```python
from build123d import *

# Parameters (mm, degrees)
F0_W     = 219.9670784175
F0_H     = 257.1922540665
F0_H_2   = 477.1593213081
F0_W_2   = 720.8151631057
F0_H_3   = 247.0399104059
F0_H_4   = 372.2520321608
F1_DEPTH = 635


with BuildPart() as f1:
    # F0 (on Front) → F1 (new body)
    with BuildSketch(Plane.XZ):
        with BuildLine():
            Line((-825.5, -1066.8), (825.5, -1066.8))
            Line((825.5, -1066.8), (825.5, 1016))
            ThreePointArc((825.5, 1016), (810.6210244843, 1051.9210244843), (774.7, 1066.8))
            Line((774.7, 1066.8), (-774.7, 1066.8))
            ThreePointArc((-774.7, 1066.8), (-810.6210244843, 1051.9210244843), (-825.5, 1016))
            Line((-825.5, 1016), (-825.5, -1066.8))
        make_face()
        with BuildLine():
            ThreePointArc((107.7734987259, 1034.2634128571), (109.6333706654, 1038.7535409176), (114.1234987259, 1040.6134128571))
            Line((114.1234987259, 1040.6134128571), (736.4234987259, 1040.6134128571))
            ThreePointArc((736.4234987259, 1040.6134128571), (740.9136267864, 1038.7535409176), (742.7734987259, 1034.2634128571))
            Line((742.7734987259, 1034.2634128571), (742.7734987259, -1035.8365871429))
            ThreePointArc((742.7734987259, -1035.8365871429), (740.9136267864, -1040.3267152035), (736.4234987259, -1042.1865871429))
            Line((736.4234987259, -1042.1865871429), (114.1234987259, -1042.1865871429))
            ThreePointArc((114.1234987259, -1042.1865871429), (109.6333706654, -1040.3267152035), (107.7734987259, -1035.8365871429))
            Line((107.7734987259, -1035.8365871429), (107.7734987259, 1034.2634128571))
        make_face(mode=Mode.SUBTRACT)
        Polygon((-787.4, -1037.2292995453), (-787.4, 1045.5707004547), (-752.9641985893, 1045.5707004547), (-32.1490354836, 1045.5707004547), (0, 1045.5707004547), (0, -1037.2292995453), (-32.1490354836, -1037.2292995453), (-252.1161139011, -1037.2292995453), (-272.5006639957, -1037.2292995453), (-734.9091768265, -1037.2292995453), (-752.9641985893, -1037.2292995453), align=None, mode=Mode.SUBTRACT)
        Polygon((-752.9641985893, 1045.5707004547), (-787.4, 1045.5707004547), (-787.4, -1037.2292995453), (-752.9641985893, -1037.2292995453), (-752.9641985893, -302.8777241707), (-752.9641985893, -59.2219047248), (-752.9641985893, 187.818005681), (-752.9641985893, 560.0700378418), (-752.9641985893, 593.9111113548), (-752.9641985893, 780.0370454788), (-752.9641985893, 813.8781785965), (-752.9641985893, 854.4874191284), (-752.9641985893, 1016.9246196747), align=None)
        with BuildLine():
            Line((-752.9641985893, -302.8777241707), (-752.9641985893, -1037.2292995453))
            Line((-752.9641985893, -1037.2292995453), (-734.9091768265, -1037.2292995453))
            Line((-734.9091768265, -1037.2292995453), (-734.9091768265, -326.3940406799))
            ThreePointArc((-734.9091768265, -326.3940406799), (-733.049304887, -321.9039126194), (-728.5591768265, -320.0440406799))
            Line((-728.5591768265, -320.0440406799), (-278.8506639957, -320.0440406799))
            ThreePointArc((-278.8506639957, -320.0440406799), (-274.3605359352, -321.9039126194), (-272.5006639957, -326.3940406799))
            Line((-272.5006639957, -326.3940406799), (-272.5006639957, -1037.2292995453))
            Line((-272.5006639957, -1037.2292995453), (-252.1161139011, -1037.2292995453))
            Line((-252.1161139011, -1037.2292995453), (-252.1161139011, -560.0699782372))
            Line((-252.1161139011, -560.0699782372), (-252.1161139011, -302.8777241707))
            Line((-252.1161139011, -302.8777241707), (-752.9641985893, -302.8777241707))
        make_face()
        with Locations((-142.1325746924, -431.4738512039)):
            Rectangle(F0_W, F0_H)
        with BuildLine():
            ThreePointArc((-238.722667098, -327.5587750435), (-236.8627951586, -323.068646983), (-232.372667098, -321.2087750435))
            Line((-232.372667098, -321.2087750435), (-50.5582434893, -321.2087750435))
            ThreePointArc((-50.5582434893, -321.2087750435), (-46.0681154287, -323.068646983), (-44.2082434893, -327.5587750435))
            Line((-44.2082434893, -327.5587750435), (-44.2082434893, -532.6683329582))
            ThreePointArc((-44.2082434893, -532.6683329582), (-46.0681154287, -537.1584610188), (-50.5582434893, -539.0183329582))
            Line((-50.5582434893, -539.0183329582), (-232.372667098, -539.0183329582))
            ThreePointArc((-232.372667098, -539.0183329582), (-236.8627951586, -537.1584610188), (-238.722667098, -532.6683329582))
            Line((-238.722667098, -532.6683329582), (-238.722667098, -327.5587750435))
        make_face(mode=Mode.SUBTRACT)
        with Locations((-142.1325746924, -798.6496388912)):
            Rectangle(F0_W, F0_H_2)
        with BuildLine():
            ThreePointArc((-238.722667098, -582.6405478477), (-236.8627951586, -578.1504197872), (-232.372667098, -576.2905478477))
            Line((-232.372667098, -576.2905478477), (-54.0525136352, -576.2905478477))
            ThreePointArc((-54.0525136352, -576.2905478477), (-49.5623855746, -578.1504197872), (-47.7025136352, -582.6405478477))
            Line((-47.7025136352, -582.6405478477), (-47.7025136352, -1017.207305336))
            ThreePointArc((-47.7025136352, -1017.207305336), (-49.5623855746, -1021.6974333965), (-54.0525136352, -1023.557305336))
            Line((-54.0525136352, -1023.557305336), (-232.372667098, -1023.557305336))
            ThreePointArc((-232.372667098, -1023.557305336), (-236.8627951586, -1021.6974333965), (-238.722667098, -1017.207305336))
            Line((-238.722667098, -1017.207305336), (-238.722667098, -582.6405478477))
        make_face(mode=Mode.SUBTRACT)
        Polygon((-752.9641985893, -59.2219047248), (-752.9641985893, -302.8777241707), (-252.1161139011, -302.8777241707), (-32.1490354836, -59.2219047248), align=None)
        with BuildLine():
            Line((-742.5824999809, -286.2870691341), (-742.5824999809, -75.7915718317))
            ThreePointArc((-742.5824999809, -75.7915718317), (-740.7226280415, -71.3014437712), (-736.2324999809, -69.4415718317))
            Line((-736.2324999809, -69.4415718317), (-71.9638137919, -69.4415718317))
            ThreePointArc((-71.9638137919, -69.4415718317), (-66.1611104022, -73.2125926982), (-67.2504119148, -80.0467266755))
            Line((-67.2504119148, -80.0467266755), (-255.8638893667, -288.972406544))
            ThreePointArc((-255.8638893667, -288.972406544), (-257.9887402532, -290.5156914705), (-260.5563342855, -291.0672171179))
            Line((-260.5563342855, -291.0672171179), (-736.2115430225, -292.6370345518))
            ThreePointArc((-736.2115430225, -292.6370345518), (-740.7152125143, -290.7846004951), (-742.5824999809, -286.2870691341))
        make_face(mode=Mode.SUBTRACT)
        Polygon((-32.1490354836, -59.2219047248), (-252.1161139011, -302.8777241707), (-32.1490354836, -302.8777241707), align=None)
        with BuildLine():
            ThreePointArc((-51.193972408, -92.0971805627), (-44.2010532487, -90.4255908565), (-40.1305705309, -96.3523354064))
            Line((-40.1305705309, -96.3523354064), (-40.1305705309, -286.3372953238))
            ThreePointArc((-40.1305705309, -286.3372953238), (-41.9621154253, -290.7989164932), (-46.4001968172, -292.6867866472))
            Line((-46.4001968172, -292.6867866472), (-219.8970689913, -294.882960675))
            ThreePointArc((-219.8970689913, -294.882960675), (-225.7637081305, -291.149120786), (-224.6908445822, -284.2783145078))
            Line((-224.6908445822, -284.2783145078), (-51.193972408, -92.0971805627))
        make_face(mode=Mode.SUBTRACT)
        with Locations((-392.5566170365, 64.2980504781)):
            Rectangle(F0_W_2, F0_H_3)
        with BuildLine():
            ThreePointArc((-744.1825866699, 169.5563005447), (-742.3227147305, 174.0464286053), (-737.8325866699, 175.9063005447))
            Line((-737.8325866699, 175.9063005447), (-48.8807489932, 175.9063005447))
            ThreePointArc((-48.8807489932, 175.9063005447), (-44.3906209326, 174.0464286053), (-42.5307489932, 169.5563005447))
            Line((-42.5307489932, 169.5563005447), (-42.5307489932, -44.1604325712))
            ThreePointArc((-42.5307489932, -44.1604325712), (-44.3906209326, -48.6505606317), (-48.8807489932, -50.5104325712))
            Line((-48.8807489932, -50.5104325712), (-737.8325866699, -50.5104325712))
            ThreePointArc((-737.8325866699, -50.5104325712), (-742.3227147305, -48.6505606317), (-744.1825866699, -44.1604325712))
            Line((-744.1825866699, -44.1604325712), (-744.1825866699, 169.5563005447))
        make_face(mode=Mode.SUBTRACT)
        with Locations((-392.5566170365, 373.9440217614)):
            Rectangle(F0_W_2, F0_H_4)
        with BuildLine():
            ThreePointArc((-740.9823536873, 542.4069570541), (-739.1224817478, 546.8970851147), (-734.6323536873, 548.7569570541))
            Line((-734.6323536873, 548.7569570541), (-48.8807489932, 548.7569570541))
            ThreePointArc((-48.8807489932, 548.7569570541), (-44.3906209326, 546.8970851147), (-42.5307489932, 542.4069570541))
            Line((-42.5307489932, 542.4069570541), (-42.5307489932, 204.6810580254))
            ThreePointArc((-42.5307489932, 204.6810580254), (-44.3906209326, 200.1909299648), (-48.8807489932, 198.3310580254))
            Line((-48.8807489932, 198.3310580254), (-734.6323536873, 198.3310580254))
            ThreePointArc((-734.6323536873, 198.3310580254), (-739.1224817478, 200.1909299648), (-740.9823536873, 204.6810580254))
            Line((-740.9823536873, 204.6810580254), (-740.9823536873, 542.4069570541))
        make_face(mode=Mode.SUBTRACT)
        Polygon((-32.1490354836, 560.0700378418), (-32.1490354836, 813.8781785965), (-752.9641985893, 813.8781785965), (-752.9641985893, 780.0370454788), (-752.9641985893, 593.9111113548), (-752.9641985893, 560.0700378418), align=None)
        with BuildLine():
            ThreePointArc((-47.4694770129, 807.8971505165), (-42.973452712, 806.0313745838), (-41.1194989413, 801.5304624804))
            Line((-41.1194989413, 801.5304624804), (-41.7140275426, 575.3059049754))
            ThreePointArc((-41.7140275426, 575.3059049754), (-43.582342696, 570.8240157377), (-48.0712380826, 568.9725971303))
            Line((-48.0712380826, 568.9725971303), (-737.8147173414, 569.7581957444))
            ThreePointArc((-737.8147173414, 569.7581957444), (-742.3090228527, 571.6295025522), (-744.1574353417, 576.1332723586))
            Line((-744.1574353417, 576.1332723586), (-743.2670072413, 801.5722312495))
            ThreePointArc((-743.2670072413, 801.5722312495), (-741.3983086815, 806.0461372166), (-736.9170567725, 807.8971505165))
            Line((-736.9170567725, 807.8971505165), (-47.4694770129, 807.8971505165))
        make_face(mode=Mode.SUBTRACT)
        Polygon((0, 1045.5707004547), (-32.1490354836, 1045.5707004547), (-32.1490354836, 813.8781785965), (-32.1490354836, 560.0700378418), (-32.1490354836, 187.818005681), (-32.1490354836, -59.2219047248), (-32.1490354836, -302.8777241707), (-32.1490354836, -560.0699782372), (-32.1490354836, -1037.2292995453), (0, -1037.2292995453), align=None)
        Polygon((-32.1490354836, 1045.5707004547), (-752.9641985893, 1045.5707004547), (-752.9641985893, 1016.9246196747), (-752.9641985893, 854.4874191284), (-752.9641985893, 813.8781785965), (-32.1490354836, 813.8781785965), align=None)
        with BuildLine():
            ThreePointArc((-47.2806287766, 1034.4494581223), (-42.790500716, 1032.5895861828), (-40.9306287766, 1028.0994581223))
            Line((-40.9306287766, 1028.0994581223), (-40.9306287766, 828.4766413002))
            ThreePointArc((-40.9306287766, 828.4766413002), (-42.7940868309, 823.9829299867), (-47.2907677906, 822.1266493947))
            Line((-47.2907677906, 822.1266493947), (-736.7300261753, 823.2274751043))
            ThreePointArc((-736.7300261753, 823.2274751043), (-741.2135984748, 825.0909250641), (-743.0698871613, 829.5774670098))
            Line((-743.0698871613, 829.5774670098), (-743.0698871613, 1028.0994581223))
            ThreePointArc((-743.0698871613, 1028.0994581223), (-741.2100152218, 1032.5895861828), (-736.7198871613, 1034.4494581223))
            Line((-736.7198871613, 1034.4494581223), (-47.2806287766, 1034.4494581223))
        make_face(mode=Mode.SUBTRACT)
    extrude(amount=F1_DEPTH)


solid = f1.part
```
For this review, take the finished solid that the model builds, in its own axes (mm). A direction names the side the tool comes from. Round coordinates to 2 decimals unless told otherwise and drop trailing zeros. Write each loop counter-clockwise with the first axis right and the second up, starting at its lowest first coordinate (ties: lowest second). Pieces come first, ordered by that corner, then holes. Notation, with made-up numbers: (-36.5, 61.5) - (-18.5, 61.5) arc R14 cw to (-18.5, 66.5) - close; hole circle Ø3 at (44, -4.5). An arc over 180 degrees is marked (long way). Answer as CSV lines item,"result". Start each with the question number.
(1) For line 1 (X direction, y = -357, z = -745.5); line 2 (X direction, y = -447, z = 474); line 3 (X direction, y = -444, z = 927), list the stretches that pass through material, from the lowest coordinate up.
(2) Machinability: for faces 5 (the flat face through (825.5, -313, -40)), 6 (the flat face through (-740.982, -313, 371)), which of the approach directions +Z, -Z, +X, -X, +Y, -Y give a long, thin tool a straight path to every point of the face, cutting with its end or side? Answer none if there is none.
(3) Add section B-B, the plane x = 247.5. State the section outline as (y, z) points, plus the area to 3 significant figures.
(4) Add section D-D, the plane y = -456. State how many separate pieces and enclosed holes the cut face has, plus the area to 3 significant figures.
(5) Mouldability with a two-part tool opening along X and no side actions: class faces 1 (the flat face through (-40.931, -313, 930)), 2 (the cylindrical face through (811.014, -313.055, 1051.524)), 3 (the flat face through (-825.5, -313, -11)), 4 (the flat face through (-12, -313, -1066.8)) as +X half, -X half, draft (parallel to the pull), parting line (faces both ways), or undercut.
(6) Add section A-A, the plane z = 500. State the section outline as (x, y) points.
(7) Add section C-C, the plane z = -695. State the section outline as (x, y) points, plus the area to 3 significant figures.
From the geometry:
1,line 1,"x = -825.5 to -734.91, -272.5 to -238.72, -47.7 to 107.77, 742.77 to 825.5"
1,line 2,"x = -825.5 to -740.98, -42.53 to 107.77, 742.77 to 825.5"
1,line 3,"x = -825.5 to -743.07, -40.93 to 107.77, 742.77 to 825.5"
2,face 5,"+Z, -Z, +X, +Y, -Y"
2,face 6,"+Y, -Y"
3,outline,"(-635, -1066.8) - (0, -1066.8) - (0, -1042.19) - (-635, -1042.19) - close; (-635, 1040.61) - (0, 1040.61) - (0, 1066.8) - (-635, 1066.8) - close"
3,area,"32,300 mm²"
4,separate pieces,"1"
4,enclosed holes,"10"
4,area,"869,000 mm²"
5,face 1,"undercut"
5,face 2,"+X half"
5,face 3,"-X half"
5,face 4,"draft"
6,outline,"(-825.5, -635) - (-740.98, -635) - (-740.98, 0) - (-825.5, 0) - close; (-42.53, -635) - (107.77, -635) - (107.77, 0) - (-42.53, 0) - close; (742.77, -635) - (825.5, -635) - (825.5, 0) - (742.77, 0) - close"
7,outline,"(-825.5, -635) - (-734.91, -635) - (-734.91, 0) - (-825.5, 0) - close; (-272.5, -635) - (-238.72, -635) - (-238.72, 0) - (-272.5, 0) - close; (-47.7, -635) - (107.77, -635) - (107.77, 0) - (-47.7, 0) - close; (742.77, -635) - (825.5, -635) - (825.5, 0) - (742.77, 0) - close"
7,area,"230,000 mm²"
